```python
from build123d import *

# Parameters (mm, degrees)
SKETCH2_W                                      = 43.5
SKETCH2_H                                      = 60
BOSS_EXTRUDE1_DEPTH                            = 2.5
SKETCH3_W                                      = 30.5
SKETCH3_H                                      = 9.5
CUT_EXTRUDE1_DEPTH                             = 38.13909665
SKETCH4_R                                      = 3.25
BOSS_EXTRUDE2_DEPTH                            = 8.5
TAP_DRILL_FOR_M3X0_5_TAP1_D                    = 2.7
FILLET1_R                                      = 5
SKETCH7_W                                      = 4
SKETCH7_H                                      = 46.25
CUT_EXTRUDE2_DEPTH                             = 1.5
CSK_FOR_8_FLAT_HEAD_MACHINE_SCREW1_D           = 4.4958
CSK_FOR_8_FLAT_HEAD_MACHINE_SCREW1_CSINK_D     = 8.4328
CSK_FOR_8_FLAT_HEAD_MACHINE_SCREW1_CSINK_ANGLE = 82


with BuildPart() as part:
    # Sketch2 → Boss-Extrude1 (new body)
    with BuildSketch(Plane(origin=(0, 0, 0), x_dir=(1, 0, 0), z_dir=(0, 1, 0))):
        Rectangle(SKETCH2_W, SKETCH2_H)
    extrude(amount=BOSS_EXTRUDE1_DEPTH)

    # Sketch3 → Cut-Extrude1 (cut, through all)
    with BuildSketch(Plane(origin=(0, 2.5, 0), x_dir=(1, 0, 0), z_dir=(0, 1, 0))):
        with Locations((0, -21)):
            Rectangle(SKETCH3_W, SKETCH3_H)
    extrude(amount=-CUT_EXTRUDE1_DEPTH, mode=Mode.SUBTRACT)

    # Sketch4 → Boss-Extrude2 (add)
    with BuildSketch(Plane(origin=(0, 2.5, 0), x_dir=(1, 0, 0), z_dir=(0, 1, 0))):
        with Locations(Location((-18.5, -21, 0), (0, 0, 180))):
            Circle(SKETCH4_R)
        with Locations(Location((18.5, -21, 0), (0, 0, 180))):
            Circle(SKETCH4_R)
    extrude(amount=BOSS_EXTRUDE2_DEPTH)

    # Tap Drill for M3x0.5 Tap1 (through all)
    with Locations(Plane(origin=(0, 11, 0), x_dir=(1, 0, 0), z_dir=(0, 1, 0))):
        with Locations((-18.5, -21), (18.5, -21)):
            Hole(TAP_DRILL_FOR_M3X0_5_TAP1_D / 2)

    # Fillet1
    fillet1_edges = [part.edges().sort_by_distance(p)[0] for p in [
        (21.75, 1.25, 30),
        (-21.75, 1.25, 30),
    ]]
    fillet(fillet1_edges, radius=FILLET1_R)

    # Sketch7 → Cut-Extrude2 (cut)
    with BuildSketch(Plane(origin=(0, 2.5, 0), x_dir=(1, 0, 0), z_dir=(0, 1, 0))):
        with Locations((0, 6.875)):
            Rectangle(SKETCH7_W, SKETCH7_H)
    extrude(amount=-CUT_EXTRUDE2_DEPTH, mode=Mode.SUBTRACT)

    # CSK for #8 Flat Head Machine Screw1 (through all)
    with Locations(Plane(origin=(0, 0, 0), x_dir=(-1, 0, 0), z_dir=(0, -1, 0))):
        with Locations((-12.7, 0.95), (-12.7, 20), (12.7, 0.95), (12.7, 20)):
            CounterSinkHole(CSK_FOR_8_FLAT_HEAD_MACHINE_SCREW1_D / 2, CSK_FOR_8_FLAT_HEAD_MACHINE_SCREW1_CSINK_D / 2, counter_sink_angle=CSK_FOR_8_FLAT_HEAD_MACHINE_SCREW1_CSINK_ANGLE)


solid = part.part
```
Geometry check sheet. Reference: the model listing, model coordinates, mm. A direction names the side the tool comes from. Coordinates: 2 decimals unless noted, no trailing zeros. Loops run counter-clockwise (first coordinate to the right, second up) from the corner with the lowest first, then second, coordinate; pieces in that order, holes last.
Item 1: Access from +Z, -Z, +X, -X, +Y, -Y to the whole of each face (thin tool, end or side, straight path). Record for faces 4 (the face through (-20.32, 1.27, 28.5)), 5 (the face through (15.25, 1, 21)), 6 (the face through (-15.921, 6.69, 19.022)), 7 (the face through (17.8, 11, 19.6)), 8 (the face through (0, 1, -7)).
Item 2: Release check for a two-part mould opening along Z. For faces 1 (the face through (20.32, 1.27, 28.5)), 2 (the face through (-19.747, 5.423, 21.517)), 3 (the face through (-12, 2.5, -5)) record: released by +Z, released by -Z, zero draft, split by the parting line, or undercut.
Item 3: Sectioned sample at D-D, the plane x = 5. Record the boundary of the cut face in (y, z), then the cut area to 3 significant figures.
Item 4: Sectioned sample at B-B, the plane z = -0.95. Record the boundary of the cut face in (x, y), then the cut area to 3 significant figures.
Item 5: Thickness scan on line 1 (Z direction, x = -12.7, y = 2.4); line 2 (Z direction, x = 18.5, y = 2.75); line 3 (X direction, y = 2.4, z = -20). Record the ranges inside material, lowest first.
Item 6: Sectioned sample at C-C, the plane y = 8.5. Record the boundary of the cut face in (x, z), then the cut area to 3 significant figures.
Item 7: Go/stop test with flat-tipped pins: pin 1 Ø4 at (x, y) = (16.5, 5.5) entering from -Z; pin 2 Ø2.5 at (x, z) = (-9.5, 25.5) entering from +Y; pin 3 Ø1.2 at (x, z) = (0, -15.5) entering from +Y. Record where each tip stops, or that it passes through.
Item 8: Sectioned sample at A-A, the plane x = 12.7. Record the boundary of the cut face in (y, z), then the cut area to 3 significant figures.
Check result:
1. face 4: +Z, -X, +Y, -Y
1. face 5: +Y, -Y
1. face 6: +Y
1. face 7: +Z, -Z, +X, -X, +Y
1. face 8: -Z, +Y
2. face 1: released by +Z
2. face 2: undercut
2. face 3: zero draft
3. outline: (0, -30) - (2.5, -30) - (2.5, 16.25) - (0, 16.25) - close; (0, 25.75) - (2.5, 25.75) - (2.5, 30) - (0, 30) - close
3. area: 126 mm2
4. outline: (-21.75, 0) - (-16.92, 0) - (-14.95, 2.26) - (-14.95, 2.5) - (-21.75, 2.5) - close; (-10.45, 2.26) - (-8.48, 0) - (8.48, 0) - (10.45, 2.26) - (10.45, 2.5) - (2, 2.5) - (2, 1) - (-2, 1) - (-2, 2.5) - (-10.45, 2.5) - close; (14.95, 2.26) - (16.92, 0) - (21.75, 0) - (21.75, 2.5) - (14.95, 2.5) - close
4. area: 71.4 mm2
5. line 1: z = -30 to -22.25, -17.75 to -3.2, 1.3 to 16.25, 25.75 to 30
5. line 2: z = 17.75 to 19.65, 22.35 to 24.25
5. line 3: x = -21.75 to -14.95, -10.45 to -2, 2 to 10.45, 14.95 to 21.75
6. outline: circle Ø6.5 at (-18.5, 21); circle Ø6.5 at (18.5, 21); hole circle Ø2.7 at (-18.5, 21); hole circle Ø2.7 at (18.5, 21)
6. area: 54.9 mm2
7. pin 1: stops at z = 17.75
7. pin 2: stops at y = 2.5
7. pin 3: stops at y = 1
8. outline: (0, -30) - (2.5, -30) - (2.5, -22.25) - (2.26, -22.25) - (0, -24.22) - close; (0, -15.78) - (2.26, -17.75) - (2.5, -17.75) - (2.5, -3.2) - (2.26, -3.2) - (0, -5.17) - close; (0, 3.27) - (2.26, 1.3) - (2.5, 1.3) - (2.5, 16.25) - (0, 16.25) - close; (0, 25.75) - (2.5, 25.75) - (2.5, 30) - (0, 30) - close
8. area: 94.9 mm2
